Could you check a few things on this model? Use its own coordinates, in mm. Face numbers are marked on the shaded views. A direction names the side the tool comes from. Coordinates: 2 decimals unless noted, no trailing zeros. Loops run counter-clockwise (first coordinate to the right, second up) from the corner with the lowest first, then second, coordinate; pieces in that order, holes last. Notation, with made-up numbers: (2, 28) -> (25, 28) arc R16 ccw to (25, 54) -> close; hole circle Ø10 at (42, 62). An arc over 180 degrees is marked (long way). One line per question, with ' | ' between items.
Autodesk Inventor part; units mm, degrees
ref_plane "YZ Plane" through (0, 0, 0) normal (1, 0, 0) x (0, 1, 0)
ref_plane "XZ Plane" through (0, 0, 0) normal (0, 1, 0) x (-1, 0, 0)
ref_plane "XY Plane" through (0, 0, 0) normal (0, 0, 1) x (1, 0, 0)
sketch "Sketch1" plane through (0, 0, 0) normal (0, 0, 1) x (1, 0, 0)
  line L0 (25.4, 12.7) -> (-25.4, 12.7)
  line L1 (-25.4, 12.7) -> (-25.4, -12.7) construction
  line L2 (-25.4, -12.7) -> (25.4, -12.7)
  line L3 (25.4, -12.7) -> (25.4, 12.7)
  line L4 (25.4, 12.7) -> (-25.4, -12.7) construction
  line L5 (-25.4, 12.7) -> (25.4, -12.7) construction
  line L6 (-25.4, -12.7) -> (-28.829, -12.7)
  line L7 (-28.829, -12.7) -> (-28.829, 12.7)
  line L8 (-28.829, 12.7) -> (-25.4, 12.7)
  point P0 (0, 0)
  dimension "d0" = 25.4
  dimension "d1" = 50.8
  dimension "d2" = 3.429
extrude "Plate1" add sketch "Sketch1" along normal blind 3.048
sketch "Sketch2" plane through (-28.829, -12.7, 3.048) normal (-1, 0, 0) x (0, -1, 0)
  line L0 (-25.4, 0) -> (0, 0)
  line L1 (0, 0) -> (0, 22.352)
  line L2 (0, 22.352) -> (-25.4, 22.352)
  line L3 (-25.4, 22.352) -> (-25.4, 0)
edge flange "Flange1" height 25.4 angle 90 thickness 3.048 bend radius 3.048 thickness toward (-1, 0, 0) relief tear relief width 3.048 relief depth 1.524 edges at (-28.829, 0, 3.048) wall of the first edge with corners at (-28.829, 12.7, 3.048) (-28.829, -12.7, 3.048) (-28.829, -12.7, 25.4) (-28.829, 12.7, 25.4)
bend "Bend1"
corner "Corner1"
sketch "Sketch3" plane through (0, 0, 3.048) normal (0, 0, 1) x (1, 0, 0)
  point P0 (0, 0)
  point P1 (0.0945, 0.5029)
hole "Hole1" at (0.0945, 0.5029, 3.048) direction (0, 0, -1) diameter 5.1054 end through all
pattern_linear "Rectangular Pattern1" count 3 spacing 12.7 along (1, 0, 0) of "Hole1" first direction both ways yes
fillet "Corner Round1" radius 3.175 4 edges at (25.4, -12.7, 1.524) (25.4, 12.7, 1.524) (-30.353, 12.7, 25.4) (-30.353, -12.7, 25.4)
equation "\"d19\" = Thickness"
equation "\"d3\" = Thickness"
equation "\"d4\" = BendReliefWidth"
equation "\"d5\" = BendReliefDepth"
equation "\"d6\" = MinimumRemnant"
equation "\"d7\" = TransitionRadius"
equation "\"d10\" = BendRadius"
equation "\"d11\" = CornerReliefSize"
equation "\"d12\" = GapSize"
equation "\"d13\" = JacobiRadiusSize"
equation "\"BendRadius\" = Thickness"
equation "\"BendReliefWidth\" = Thickness"
equation "\"BendReliefDepth\" = 0.5 * Thickness"
equation "\"CornerReliefSize\" = 4 * Thickness"
equation "\"MinimumRemnant\" = 2 * Thickness"
equation "\"TransitionRadius\" = BendRadius"
equation "\"JacobiRadiusSize\" = BendRadius"
equation "\"GapSize\" = Thickness"
properties part number "MOUNT,FLANGE,BELLYPAN" material "Steel, Alloy"
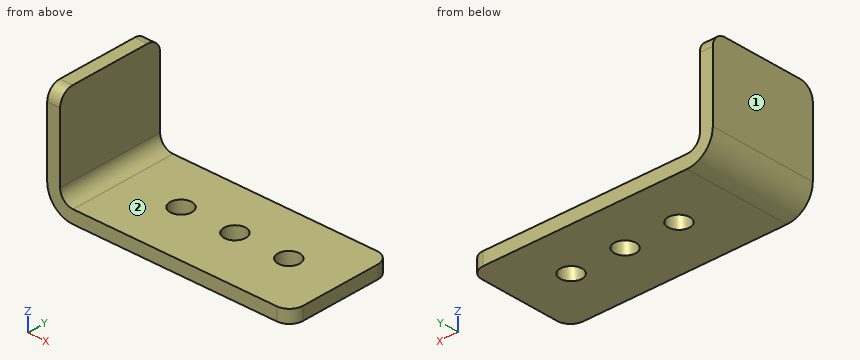
1) On a 3-axis mill with a long thin cutter (end or side, diameter ignored), from which of +Z, -Z, +X, -X, +Y, -Y can I reach the whole of each face in a straight line? I mean the marked faces 1 and 2. Say none if no direction works.
Data:
face 1: +Z, -Z, -X, +Y, -Y | face 2: +Z, +X, +Y, -Y
2) If we section it at A-A on y = -1.25: Please give me the cut outline in (x, z), and give its area (3 significant figures).
Data:
outline: (-31.88, 6.1) arc R6.1 ccw to (-25.78, 0) -> (-14.46, 0) -> (-14.46, 3.05) -> (-25.78, 3.05) arc R3.05 cw to (-28.83, 6.1) -> (-28.83, 25.4) -> (-31.88, 25.4) -> close; (-10.75, 0) -> (-1.76, 0) -> (-1.76, 3.05) -> (-10.75, 3.05) -> close; (1.95, 0) -> (10.94, 0) -> (10.94, 3.05) -> (1.95, 3.05) -> close; (14.65, 0) -> (25.4, 0) -> (25.4, 3.05) -> (14.65, 3.05) -> close | area: 203 mm²
3) If we section it at D-D on y = 1.5: Please give me the cut outline in (x, z), and give its area (3 significant figures).
Data:
outline: (-31.88, 6.1) arc R6.1 ccw to (-25.78, 0) -> (-14.96, 0) -> (-14.96, 3.05) -> (-25.78, 3.05) arc R3.05 cw to (-28.83, 6.1) -> (-28.83, 25.4) -> (-31.88, 25.4) -> close; (-10.26, 0) -> (-2.26, 0) -> (-2.26, 3.05) -> (-10.26, 3.05) -> close; (2.44, 0) -> (10.44, 0) -> (10.44, 3.05) -> (2.44, 3.05) -> close; (15.14, 0) -> (25.4, 0) -> (25.4, 3.05) -> (15.14, 3.05) -> close | area: 194 mm²
4) I need wall thicknesses on line 1 along Z through (x, y) = (21, -9.75); line 2 along X through (y, z) = (7.25, 12.75); line 3 along X through (y, z) = (6.5, 3.5). Which ranges of each line are inside material? Lowest first, please. Write a range as from..to.
Data:
line 1: 0..3.05 | line 2: -31.88..-28.83 | line 3: -31.3..-27.38
5) If we section it at C-C on z = 12.25: Please give me the cut outline in (x, y).
Data:
outline: (-31.88, -12.7) -> (-28.83, -12.7) -> (-28.83, 12.7) -> (-31.88, 12.7) -> close
6) If we section it at B-B on x = -7: Please give me the cut outline in (y, z), and give its area (3 significant figures).
Data:
outline: (-12.7, 0) -> (12.7, 0) -> (12.7, 3.05) -> (-12.7, 3.05) -> close | area: 77.4 mm²
7) I'm going to push flat-ended pins straight in: pin 1 Ø3 at (x, y) = (-12.61, 0.5) entering from -Z; pin 2 Ø6 at (x, y) = (11.5, -1.5) entering from +Z; pin 3 Ø2 at (y, z) = (-6, 4.5) entering from +X; pin 4 Ø5 at (x, y) = (-25, -6.5) entering from +Z. Where does each tip first touch, or does it pass through?
Data:
pin 1: through | pin 2: z = 3.05 | pin 3: x = -27.38 | pin 4: z = 3.58
